```python
from build123d import *

# Parameters (mm, degrees)
ESQUISSE1_W                = 189
ESQUISSE1_H                = 125
BOSS_EXTRU_1_DEPTH         = 10
ESQUISSE2_W                = 30
ESQUISSE2_H                = 15
ENL_V_MAT_EXTRU_1_DEPTH    = 10
ESQUISSE3_W                = 10
ESQUISSE3_H                = 10
ENL_V_MAT_EXTRU_2_DEPTH    = 10
R_P_TITION_LIN_AIRE1_COUNT = 8
R_P_TITION_LIN_AIRE1_PITCH = 20
ESQUISSE4_R                = 5
BOSS_EXTRU_2_DEPTH         = 25
ESQUISSE5_R                = 5
BOSS_EXTRU_4_DEPTH         = 25


with BuildPart() as part:
    # Esquisse1 → Boss.-Extru.1 (new body)
    with BuildSketch(Plane(origin=(0, 0, 0), x_dir=(1, 0, 0), z_dir=(0, 1, 0))):
        with Locations((-94.5, 62.5)):
            Rectangle(ESQUISSE1_W, ESQUISSE1_H)
    extrude(amount=BOSS_EXTRU_1_DEPTH)

    # Esquisse2 → Enlèv. mat.-Extru.1 (cut)
    with BuildSketch(Plane(origin=(0, 10, 0), x_dir=(1, 0, 0), z_dir=(0, 1, 0))):
        with Locations((-174, 117.5)):
            Rectangle(ESQUISSE2_W, ESQUISSE2_H)
        with Locations((-174, 7.5)):
            Rectangle(ESQUISSE2_W, ESQUISSE2_H)
    extrude(amount=-ENL_V_MAT_EXTRU_1_DEPTH, mode=Mode.SUBTRACT)

    # Esquisse3 → Enlèv. mat.-Extru.2 (cut)
    with BuildSketch(Plane(origin=(0, 10, 0), x_dir=(1, 0, 0), z_dir=(0, 1, 0))):
        with Locations((-144, 120)):
            Rectangle(ESQUISSE3_W, ESQUISSE3_H)
        with Locations((-144, 5)):
            Rectangle(ESQUISSE3_W, ESQUISSE3_H)
    enl_v_mat_extru_2 = extrude(amount=-ENL_V_MAT_EXTRU_2_DEPTH, mode=Mode.SUBTRACT)

    # Répétition linéaire1: Enlèv. mat.-Extru.2 ×8
    with Locations(*[(i * R_P_TITION_LIN_AIRE1_PITCH, 0, 0) for i in range(1, R_P_TITION_LIN_AIRE1_COUNT)]):
        add(enl_v_mat_extru_2, mode=Mode.SUBTRACT)

    # Esquisse4 → Boss.-Extru.2 (add)
    with BuildSketch(Plane.XY.offset(-15)):
        with Locations((-184, 5)):
            Circle(ESQUISSE4_R)
    extrude(amount=BOSS_EXTRU_2_DEPTH)

    # Esquisse5 → Boss.-Extru.4 (add)
    with BuildSketch(Plane(origin=(0, 0, -110), x_dir=(-1, 0, 0), z_dir=(0, 0, -1))):
        with Locations((184, 5)):
            Circle(ESQUISSE5_R)
    extrude(amount=BOSS_EXTRU_4_DEPTH)


solid = part.part
```
For this review, take the finished solid that the model builds, in its own axes (mm). A direction names the side the tool comes from. Give positions to 0.01 mm unless a question says otherwise; leave off trailing zeros. One line per item, written item: value.
1) For faces 1 (the flat face through (-29, 5, -120)), 2 (the flat face through (-54, 5, -125)), 3 (the cylindrical face through (-188, 2, -3)), 4 (the flat face through (-89, 5, -5)), list the 3-axis set-ups (+Z, -Z, +X, -X, +Y, -Y) from which the entire face can be reached by the end or side of a thin tool; tool diameter is ignored.
Results are:
face 1: -Z, +Y, -Y
face 2: -Z, +X, +Y, -Y
face 3: +Z
face 4: +Z, +Y, -Y
2) For P1, Ø3, axis at y = 3, z = -6, coming from the -X side; P2, Ø5, axis at x = -91.5, y = 3.5, coming from the +Z side; P3, Ø5, axis at y = 4.5, z = -118, coming from the +X side; P4, Ø1, axis at x = -88, z = -119, coming from the -Y side, all flat-tipped, find the tip position at first contact; note any pin that passes through.
Results are:
P1: stops at x = -188.97
P2: stops at z = 0
P3: stops at x = -9
P4: passes through
3) The part is to be moulded in two halves that separate along X. For faces 5 (the flat face through (-64, 5, -115)), 6 (the flat face through (-188, 1, -15)), 7 (the flat face through (-39, 5, -5)), say which applies: +X half, -X half, draft (parallel to the pull), parting line (faces both ways), or undercut.
Results are:
face 5: undercut
face 6: draft
face 7: undercut
4) For line 1 (Z direction, x = -161, y = 6.5); line 2 (Z direction, x = -62.5, y = 9); line 3 (X direction, y = 3, z = -12), list the stretches that pass through material, from the lowest coordinate up. Write a range as from..to.
Results are:
line 1: z = -110..-15
line 2: z = -115..-10
line 3: x = -188.58..-179.42, -159..0
